Can you work these out from the model? Positions are in its coordinate system, mm. Face numbers are marked on the shaded views. Round coordinates to 2 decimals unless told otherwise and drop trailing zeros. Write each loop counter-clockwise with the first axis right and the second up, starting at its lowest first coordinate (ties: lowest second). Pieces come first, ordered by that corner, then holes. Notation, with made-up numbers: (35.25, 36.5) - (57.25, 36.5) arc R11 ccw to (57.25, 48.5) - close; hole circle Ø5 at (-12.75, 11). An arc over 180 degrees is marked (long way). One line per item, written item: value. Start each with the question number.
(1) Thinking about a two-plate mould opening in Z: for the marked faces 1 and 2, which applies, +Z half, -Z half, draft (parallel to the pull), parting line (faces both ways), or undercut?
(2) I want a section at C-C on z = -46. List the corners of the cut face in (x, y) for me.
(3) I want a section at D-D on x = 84.25. List the corners of the cut face in (y, z) for me, plus the area to 3 significant figures.
(4) I want a section at A-A on z = -60.5. List the corners of the cut face in (x, y) for me.
(5) I'm going to push flat-ended pins straight in: pin 1 Ø1 at (x, z) = (70, -70) entering from -Y; pin 2 Ø5.5 at (x, z) = (60.5, -111) entering from +Y; pin 3 Ø2.5 at (x, z) = (60.5, -111) entering from +Y; pin 4 Ø10 at (x, z) = (35.5, -27.5) entering from -Y. Where does each tip first touch, or does it pass through?
(6) If I drill on L1, parallel to Z at x = 60.5, y = 0.75; L2, parallel to Z at x = 60.5, y = 2.4; L3, parallel to X at y = 0.85, z = -111, over which ranges is the centre line in solid material (lowest first)? Write a range as from..to.
(7) I want a section at B-B on x = 60.5. List the corners of the cut face in (y, z) for me, plus the area to 3 significant figures.
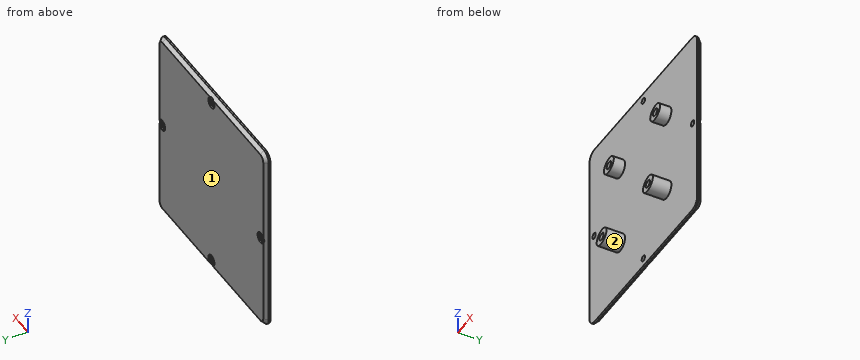
from build123d import *

# Parameters (mm, degrees)
BOSS_EXTRUDE1_DEPTH                                  = 3
CHAMFER1_SIZE                                        = 2
CBORE_FOR_M3_CROSS_RECESS_PAN_HEAD_SCREW_D           = 3.4
CBORE_FOR_M3_CROSS_RECESS_PAN_HEAD_SCREW_DEPTH       = 5
CBORE_FOR_M3_CROSS_RECESS_PAN_HEAD_SCREW_CBORE_D     = 6.2
CBORE_FOR_M3_CROSS_RECESS_PAN_HEAD_SCREW_CBORE_DEPTH = 1
CBORE_FOR_M3_CROSS_RECESS_PAN_HEAD_SCREW_TIP         = 1.021463052
SKETCH10_R                                           = 5
BOSS_EXTRUDE4_DEPTH                                  = 11
CUT_EXTRUDE4_REACH                                   = 165.994
SKETCH12_R                                           = 2.2
CUT_EXTRUDE5_DEPTH                                   = 6


with BuildPart() as part:
    # Sketch1 → Boss-Extrude1 (new body)
    with BuildSketch(Plane(origin=(0, 0, 0), x_dir=(1, 0, 0), z_dir=(0, 1, 0))):
        with BuildLine():
            Line((10.3, 5.3), (110.7, 5.3))
            ThreePointArc((110.7, 5.3), (114.235533906, 6.764466094), (115.7, 10.3))
            Line((115.7, 10.3), (115.7, 110.7))
            ThreePointArc((115.7, 110.7), (114.235533906, 114.235533906), (110.7, 115.7))
            Line((110.7, 115.7), (10.3, 115.7))
            ThreePointArc((10.3, 115.7), (6.764466094, 114.235533906), (5.3, 110.7))
            Line((5.3, 110.7), (5.3, 10.3))
            ThreePointArc((5.3, 10.3), (6.764466094, 6.764466094), (10.3, 5.3))
        make_face()
    extrude(amount=BOSS_EXTRUDE1_DEPTH)

    # Chamfer1
    chamfer1_edges = [part.edges().sort_by_distance(p)[0] for p in [
        (115.7, 3, -60.5),
        (114.235533906, 3, -6.764466094),
        (60.5, 3, -5.3),
        (6.764466094, 3, -6.764466094),
        (5.3, 3, -60.5),
        (6.764466094, 3, -114.235533906),
        (60.5, 3, -115.7),
        (114.235533906, 3, -114.235533906),
    ]]
    chamfer(chamfer1_edges, length=CHAMFER1_SIZE)

    # CBORE for M3 Cross Recess Pan Head Screw1
    with Locations(Plane(origin=(0, 3, 0), x_dir=(1, 0, 0), z_dir=(0, 1, 0))):
        with Locations((60.5, 111), (10, 60.5), (60.5, 10), (111, 60.5)):
            CounterBoreHole(CBORE_FOR_M3_CROSS_RECESS_PAN_HEAD_SCREW_D / 2, CBORE_FOR_M3_CROSS_RECESS_PAN_HEAD_SCREW_CBORE_D / 2, CBORE_FOR_M3_CROSS_RECESS_PAN_HEAD_SCREW_CBORE_DEPTH, depth=CBORE_FOR_M3_CROSS_RECESS_PAN_HEAD_SCREW_DEPTH)
            with Locations((0, 0, -(CBORE_FOR_M3_CROSS_RECESS_PAN_HEAD_SCREW_DEPTH + CBORE_FOR_M3_CROSS_RECESS_PAN_HEAD_SCREW_TIP / 2))):  # 118° drill point
                Cone(0, CBORE_FOR_M3_CROSS_RECESS_PAN_HEAD_SCREW_D / 2, CBORE_FOR_M3_CROSS_RECESS_PAN_HEAD_SCREW_TIP, mode=Mode.SUBTRACT)

    # Sketch10 → Boss-Extrude4 (add)
    with BuildSketch(Plane.XZ):
        with Locations(Location((36.75, -36.764162159, 0), (0, 0, 270))):
            Circle(SKETCH10_R)
        with Locations(Location((36.75, -84.264162159, 0), (0, 0, 270))):
            Circle(SKETCH10_R)
        with Locations(Location((84.25, -84.264162159, 0), (0, 0, 270))):
            Circle(SKETCH10_R)
        with Locations(Location((84.25, -36.764162159, 0), (0, 0, 270))):
            Circle(SKETCH10_R)
    extrude(amount=BOSS_EXTRUDE4_DEPTH)

    # Cut-Extrude4: up to this face of the body (flat: up to its plane)
    cut_extrude4_end = Plane(part.part.faces().sort_by_distance((115.7, 0.5, -60.5))[0])
    # Sketch11 → Cut-Extrude4 (cut, up to the picked face)
    with BuildSketch(Plane(origin=(0, 0, 0), x_dir=(0, 0, -1), z_dir=(1, 0, 0)), mode=Mode.PRIVATE) as cut_extrude4_sk1:
        Polygon((31.764162159, -11), (31.764162159, -6), (89.264162159, -11), align=None)
    cut_extrude4_tool1 = split(extrude(cut_extrude4_sk1.sketch, amount=CUT_EXTRUDE4_REACH, mode=Mode.PRIVATE), bisect_by=cut_extrude4_end, keep=Keep.BOTH, mode=Mode.PRIVATE)
    add(cut_extrude4_tool1.solids().sort_by(Axis((0, -9.333333, -50.930829), (1, 0, 0)))[0], mode=Mode.SUBTRACT)

    # Sketch12 → Cut-Extrude5 (cut)
    with BuildSketch(Plane(origin=(0, -3.213599513, 0.279443436), x_dir=(1, 0, 0), z_dir=(0, -0.9962405881956831, 0.08662961636484202))):
        with Locations(Location((84.25, -84.862639202, 0), (0, 0, 270))):
            Circle(SKETCH12_R)
        with Locations(Location((36.75, -84.862639202, 0), (0, 0, 270))):
            Circle(SKETCH12_R)
        with Locations(Location((36.75, -37.183393282, 0), (0, 0, 270))):
            Circle(SKETCH12_R)
        with Locations(Location((84.25, -37.183393282, 0), (0, 0, 270))):
            Circle(SKETCH12_R)
    extrude(amount=-CUT_EXTRUDE5_DEPTH, mode=Mode.SUBTRACT)


solid = part.part
Established:
1. face 1: draft
1. face 2: undercut
2. outline: (5.3, 0) - (115.7, 0) - (115.7, 1) - (113.7, 3) - (7.3, 3) - (5.3, 1) - close
3. outline: (-11, -89.26) - (0, -89.26) - (0, -115.7) - (1, -115.7) - (3, -113.7) - (3, -7.3) - (1, -5.3) - (0, -5.3) - (0, -31.76) - (-6, -31.76) - (-6.24, -34.57) - (-0.27, -35.09) - (-0.65, -39.48) - (-6.63, -38.96) - (-6.87, -41.76) - (0, -41.76) - (0, -79.26) - (-10.13, -79.26) - (-10.37, -82.07) - (-4.4, -82.59) - (-4.78, -86.98) - (-10.76, -86.46) - close
3. area: 444 mm2
4. outline: (5.3, 0) - (8.3, 0) - (8.3, 2) - (6.9, 2) - (6.9, 2.6) - (5.3, 1) - close; (11.7, 0) - (109.3, 0) - (109.3, 2) - (107.9, 2) - (107.9, 3) - (13.1, 3) - (13.1, 2) - (11.7, 2) - close; (112.7, 0) - (115.7, 0) - (115.7, 1) - (114.1, 2.6) - (114.1, 2) - (112.7, 2) - close
5. pin 1: y = 0
5. pin 2: y = 2
5. pin 3: through
5. pin 4: y = -6.06
6. L1: -115.7..-112.7, -109.3..-11.7, -8.3..-5.3
6. L2: -114.3..-114.1, -107.9..-13.1, -6.9..-6.7
6. L3: 5.31..58.8, 62.2..115.69
7. outline: (0, -115.7) - (1, -115.7) - (2.6, -114.1) - (2, -114.1) - (2, -112.7) - (0, -112.7) - close; (0, -109.3) - (2, -109.3) - (2, -107.9) - (3, -107.9) - (3, -13.1) - (2, -13.1) - (2, -11.7) - (0, -11.7) - close; (0, -8.3) - (2, -8.3) - (2, -6.9) - (2.6, -6.9) - (1, -5.3) - (0, -5.3) - close
7. area: 301 mm2
